Read the model definition and answer for the solid it produces. Units are mm, in the model's axes. Face numbers are marked on the shaded views. Coordinates: 2 decimals unless noted, no trailing zeros. Loops run counter-clockwise (first coordinate to the right, second up) from the corner with the lowest first, then second, coordinate; pieces in that order, holes last. Notation, with made-up numbers: (-28.75, -8.5) - (1.25, -8.5) arc R20 cw to (1.25, 14.5) - close; hole circle Ø10 at (33.5, 68). An arc over 180 degrees is marked (long way). One line per item, written item: value. Start each with the question number.
from build123d import *

# Parameters (mm, degrees)
F0_W     = 50
F0_H     = 50
F1_DEPTH = 26
F3_DEPTH = 50.001


with BuildPart() as f1:
    # F0 (on Top) → F1 (new body)
    with BuildSketch(Plane.XY):
        Rectangle(F0_W, F0_H)
    extrude(amount=F1_DEPTH)

    # F2 (on face) → F3 (cut, through all)
    with BuildSketch(Plane.XZ.offset(25)):
        with BuildLine():
            ThreePointArc((6.792214, 26), (19.667063, 20.667063), (25, 7.792214))
            Line((25, 7.792214), (25, 26))
            Line((25, 26), (6.792214, 26))
        make_face()
        with BuildLine():
            Line((-25, 26), (-25, 7.792214))
            ThreePointArc((-25, 7.792214), (-19.667063, 20.667063), (-6.792214, 26))
            Line((-6.792214, 26), (-25, 26))
        make_face()
    extrude(amount=-F3_DEPTH, mode=Mode.SUBTRACT)


solid = f1.part
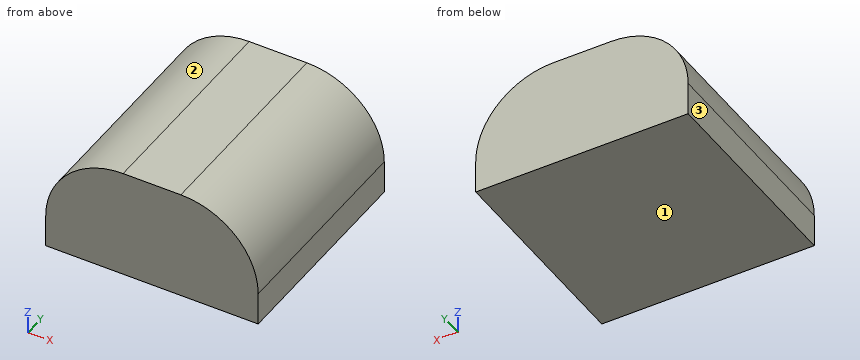
1) Straight lines are drawn through the part: L1, parallel to X at y = 6, z = 8.5; L2, parallel to X at y = 14.5, z = 24.5; L3, parallel to Z at x = 7.5, y = -21.5. For each, find the intervals that lie inside material, in ascending order.
2) Section A-A, the plane y = 9.5 is taken. Determine the outline of the cut face in (x, z), and give its area (3 significant figures).
3) Section B-B, the plane x = 12.5 is taken. Determine the outline of the cut face in (y, z).
4) Flat-ended cylindrical pins translate along their axes: P1, Ø1.5, axis at x = -14, y = 0, coming from the +Z side; P2, Ø6, axis at x = -13.5, y = 11.5, coming from the +Z side; P3, Ø5, axis at x = 17, y = -9.5, coming from the +Z side. Find the tip coordinate at first contact, or state that the pin passes through.
5) Determine the mould class of the marked faces 1, 2 and 3 for opening direction Z: released by +Z, released by -Z, zero draft, split by the parting line, or undercut.
6) Section C-C, the plane z = 14 is taken. Determine the outline of the cut face in (x, y), and give its area (3 significant figures).
Answer below:
1. L1: -24.99 to 24.99
1. L2: -14.03 to 14.03
1. L3: 0 to 25.99
2. outline: (-25, 0) - (25, 0) - (25, 7.79) arc R18.21 ccw to (6.79, 26) - (-6.79, 26) arc R18.21 ccw to (-25, 7.79) - close
2. area: 1,160 mm2
3. outline: (-25, 0) - (25, 0) - (25, 25.08) - (-25, 25.08) - close
4. P1: z = 24.82
4. P2: z = 25.62
4. P3: z = 24.29
5. face 1: released by -Z
5. face 2: released by +Z
5. face 3: zero draft
6. outline: (-23.91, -25) - (23.91, -25) - (23.91, 25) - (-23.91, 25) - close
6. area: 2,390 mm2
